CAD build for the part. Positions are in the model's coordinates, mm. A direction names the side the tool comes from. Give positions to 0.01 mm unless a question says otherwise; leave off trailing zeros. Order: outer loops, then holes, each group sorted by start corner. A loop starts at its lowest first (then second) coordinate and runs counter-clockwise, first axis right, second up. Notation, with made-up numbers: (53, -17.75) -> (112, -17.75) arc R9 ccw to (112, -0.75) -> close; hole circle Ø3 at (-33.75, -24). An arc over 180 degrees is marked (long way). Answer as CSV lines item,"result".
Autodesk Inventor part; units mm, degrees
ref_plane "YZ Plane" through (0, 0, 0) normal (1, 0, 0) x (0, 1, 0)
ref_plane "XZ Plane" through (0, 0, 0) normal (0, 1, 0) x (-1, 0, 0)
ref_plane "XY Plane" through (0, 0, 0) normal (0, 0, 1) x (1, 0, 0)
sketch "Esboço1" plane through (0, 0, 0) normal (0, 1, 0) x (-1, 0, 0)
  line L0 (0, 0) -> (0, -16)
  line L1 (0, -16) -> (-34.5, -16)
  line L2 (-34.5, -16) -> (-34.5, 0)
  line L3 (-34.5, 0) -> (0, 0)
  line L4 (-3.5, -14.5) -> (-16.5, -14.5)
  line L5 (-16.5, -14.5) -> (-16.5, -1.5)
  line L6 (-16.5, -1.5) -> (-3.5, -1.5)
  line L7 (-18, -14.5) -> (-33, -14.5)
  line L8 (-33, -14.5) -> (-33, -1.5)
  line L9 (-33, -1.5) -> (-18, -1.5)
  line L10 (-18, -1.5) -> (-18, -14.5)
  line L11 (-3.5, -14.5) -> (-3.5, -12)
  line L12 (-3.5, -12) -> (-1.5, -12)
  line L13 (-1.5, -12) -> (-1.5, -4)
  line L14 (-1.5, -4) -> (-3.5, -4)
  line L15 (-3.5, -4) -> (-3.5, -1.5)
  point P0 (-34.5, -8)
  dimension "d0" = 13
  dimension "d1" = 13
  dimension "d2" = 15
  dimension "d3" = 13
  dimension "d4" = 8
  dimension "d5" = 2.5
  dimension "d6" = 1.5
  dimension "d7" = 1.5
  dimension "d8" = 2
  dimension "d9" = 1.5
  dimension "d10" = 1.5
  dimension "d11" = 1.5
extrude "Extrusão1" add sketch "Esboço1" along normal blind 1.5 contours L4 L5 L6 L15 L14 L13 L12 L11 | L7 L8 L9 L10
extrude "Extrusão2" add sketch "Esboço1" along normal blind 20
sketch "Esboço2" plane through (0, 0, -16) normal (-1, 0, 0) x (0, 0, 1)
  line L0 (12, 20) -> (4, 20)
  line L1 (8, 20) -> (8, 0)
  line L2 (0, 0) -> (0, 20)
  circle A0 centre (5.45, 8) radius 0.5
  circle A1 centre (10.55, 8) radius 0.5
  line L3 (0, 0) -> (16, 0)
  dimension "d23" = 8
extrude "Extrusão3" cut sketch "Esboço2" against normal blind 10
sketch "Esboço3" plane through (34.5, 0, 0) normal (1, 0, 0) x (0, 0, -1)
  line L0 (0, 20) -> (16, 20)
  line L1 (8, 20) -> (8, 0)
  circle A0 centre (6.75, 8) radius 0.5
  circle A1 centre (9.25, 8) radius 0.5
  line L2 (0, 0) -> (16, 0)
  line L3 (11, 16) -> (11, 8)
  line L4 (11, 8) -> (5, 8)
  line L5 (5, 8) -> (5, 16)
  circle A2 centre (5, 12) radius 1.5
  circle A3 centre (11, 12) radius 1.5
  dimension "d26" = 1
  dimension "d27" = 1
  dimension "d28" = 8
  dimension "d29" = 8
  dimension "d30" = 1.25
  dimension "d31" = 1.25
  dimension "d78" = 3
  dimension "d79" = 3
  dimension "d80" = 3
  dimension "d81" = 3
extrude "Extrusão4" cut sketch "Esboço3" against normal blind 10 contours L4 A0 | A1 L4 | L4 A1 | A0 L4
sketch "Esboço4" plane through (18, 1.5, -14.5) normal (1, 0, 0) x (0, 0, -1)
  line L0 (-14.5, -1.5) -> (1.5, -1.5)
  line L1 (-6.5, -1.5) -> (-6.5, 18.5)
  line L2 (0, 18.5) -> (-13, 18.5)
  circle A0 centre (-6.5, 6.5) radius 2.5
  line L3 (0, 0) -> (-13, 0)
  dimension "d40" = 5
  dimension "d42" = 6.5
extrude "Extrusão5" cut sketch "Esboço4" against normal blind 10
sketch "Esboço6" plane through (0, 20, 0) normal (0, 1, 0) x (1, 0, 0)
  line L0 (0, 0) -> (34.5, 0)
  line L1 (0, 0) -> (16.5, 0)
  line L2 (0, 0) -> (16.5, 0) construction
  line L3 (16.5, 14.5) -> (16.5, 1.5)
  line L4 (16.5, 0) -> (16.5, 1.5)
  line L5 (16.5, 1.5) -> (3.5, 1.5)
  line L6 (16.5, 1.5) -> (3.5, 1.5)
  line L7 (3.5, 1.5) -> (3.5, 4)
  line L8 (3.5, 1.5) -> (3.5, 4)
  line L9 (3.5, 4) -> (1.5, 4)
  line L10 (3.5, 4) -> (1.5, 4)
  line L11 (1.5, 4) -> (1.5, 12)
  line L12 (1.5, 12) -> (3.5, 12)
  line L13 (1.5, 12) -> (3.5, 12)
  line L14 (3.5, 12) -> (3.5, 14.5)
  line L15 (3.5, 12) -> (3.5, 14.5)
  line L16 (3.5, 14.5) -> (16.5, 14.5)
  line L17 (3.5, 14.5) -> (16.5, 14.5)
  line L18 (16.5, 14.5) -> (16.5, 16)
  line L19 (34.5, 16) -> (0, 16)
  line L20 (0, 16) -> (0, 0)
  line L21 (0, 16.0004) -> (0, 0)
  dimension "d66" = 16.5
  dimension "d67" = 0
extrude "Extrusão8" add sketch "Esboço6" along normal blind 3.5 contours L20 L19 L18 L16 L14 L12 L11 L9 L7 L5 L4 L0
sketch "Sketch8" plane through (0, 23.5, 0) normal (0, 1, 0) x (1, 0, 0)
  line L0 (3.5, 1.5) -> (16.5, 1.5)
  line L1 (6, 1.5) -> (6, -0.5)
  line L2 (6, -0.5) -> (14, -0.5)
  line L3 (14, -0.5) -> (14, 1.5)
  line L4 (16.5, 1.5) -> (14, 1.5)
  line L5 (3.5, 1.5) -> (3.5, -2)
  line L6 (3.5, -2) -> (16.5, -2)
  line L7 (16.5, -2) -> (16.5, 1.5)
  line L8 (0, 0) -> (34.5, 0)
  point P0 (6, 0)
  point P1 (14, 0)
  dimension "d86" = 8
  dimension "d87" = 2.5
  dimension "d88" = 2
  dimension "d89" = 2
  dimension "d90" = 3.5
extrude "Extrusion12" add sketch "Sketch8" against normal up to surface (23.5 mm away) contours L0 L1 L8 L5 | L8 L1 L2 L3 L7 L6 L5 | L0 L7 L8 L3
extrude "Extrusion13" cut sketch "Sketch8" against normal blind 22 contours L0 L3 L8 L1
sketch "Sketch9" plane through (0, 23.5, 0) normal (0, 1, 0) x (1, 0, 0)
  line L0 (34.5, 16) -> (0, 16)
  line L1 (0, 0) -> (3.5, 0)
  line L2 (0, 16) -> (1.5, 16)
  line L3 (1.5, 16) -> (1.5, 0)
  line L4 (1.5, 0) -> (0, 0)
  line L5 (0, 0) -> (0, 16)
  line L6 (3.5, 12) -> (1.5, 12)
  line L7 (3.5, 1.5) -> (3.5, 4)
  line L8 (3.5, 12) -> (3.5, 4)
  dimension "d95" = 1.5
extrude "Extrusion14" cut sketch "Sketch9" against normal through all
sketch "Sketch10" plane through (0, 23.5, 0) normal (0, 1, 0) x (1, 0, 0)
  line L0 (3.5, 14.5) -> (3.5, 12)
  line L1 (1.5, 12) -> (1.5, 4)
  line L2 (3.5, 12) -> (1.5, 12)
  line L3 (1.5, 12) -> (1.5, 4)
  line L4 (1.5, 4) -> (3.5, 4)
  line L5 (3.5, 4) -> (3.5, 12)
  point P0 (0, 0)
extrude "Extrusion15" add sketch "Sketch10" against normal up to surface (22 mm away)
sketch "Sketch11" plane through (0, 0, 0) normal (0, -1, 0) x (1, 0, 0)
  line L0 (6, 0) -> (14, 0)
  line L1 (6, 0.5) -> (14, 0.5)
  line L2 (6, 0) -> (14, 0)
  line L3 (14, 0) -> (14, 0.5)
  line L4 (14, 0.5) -> (6, 0.5)
  line L5 (6, 0.5) -> (6, 0)
  point P0 (0, 0)
extrude "Extrusion16" add sketch "Sketch11" against normal blind 1.5
sketch "Sketch12" plane through (0, 23.5, 0) normal (0, 1, 0) x (1, 0, 0)
  line L0 (1.5, 16) -> (1.5, 0)
  line L1 (3.5, -2) -> (3.5, 0)
  line L2 (1.5, 0) -> (3.5, 0)
  line L3 (3.5, 0) -> (3.5, -2)
  line L4 (3.5, -2) -> (1.5, -2)
  line L5 (1.5, -2) -> (1.5, 0)
  point P0 (0, 0)
extrude "Extrusion17" add sketch "Sketch12" against normal up to surface (23.5 mm away)
sketch "Sketch13" plane through (16.5, 0, 2) normal (0, 0, 1) x (1, 0, 0)
  line L0 (-13, 23.5) -> (0, 23.5)
  line L1 (-6.5, 23.5) -> (-6.5, 0)
  circle A0 centre (-3.95, 8) radius 0.75
  circle A1 centre (-9.05, 8) radius 0.75
  line L2 (0, 0) -> (-15, 0)
  line L3 (0, 23.5) -> (0, 0)
  point P0 (-16.5, 0)
  dimension "d104" = 1.5
  dimension "d105" = 1.5
  dimension "d106" = 8
  dimension "d107" = 8
  dimension "d108" = 6.5
  dimension "d109" = 2.55
  dimension "d110" = 2.55
extrude "Extrusion18" cut sketch "Sketch13" against normal blind 10 contours A0 | A1
properties part number "Base_3DPrint"
1) Band-saw the part on B-B, the plane y = 16.5. Write the cut outline in (x, z), then the cut area to 3 significant figures.
Data:
outline,"(1.5, -16) -> (34.5, -16) -> (34.5, 0) -> (16.5, 0) -> (16.5, 2) -> (1.5, 2) -> close; hole (3.5, -14.5) -> (16.5, -14.5) -> (16.5, -1.5) -> (14, -1.5) -> (14, 0.5) -> (6, 0.5) -> (6, -1.5) -> (3.5, -1.5) -> close; hole (18, -14.5) -> (33, -14.5) -> (33, -1.5) -> (18, -1.5) -> close"
area,"178 mm2"
2) Pin check, flat tips, straight feed: P1, Ø5, axis at x = 28, z = -1, coming from the +Y side; P2, Ø5, axis at x = 9, z = -2.5, coming from the +Y side; P3, Ø1.6, axis at y = 21.5, z = -15, coming from the +X side. Stop position of each tip, or through.
Data:
P1,"stops at y = 20"
P2,"stops at y = 1.5"
P3,"stops at x = 16.5"
3) Band-saw the part on A-A, the plane x = 7.45. Write the cut outline in (y, z).
Data:
outline,"(0, -16) -> (23.5, -16) -> (23.5, -14.5) -> (1.5, -14.5) -> (1.5, 0.5) -> (7.25, 0.5) -> (7.25, 2) -> (0, 2) -> close; (8.75, 0.5) -> (23.5, 0.5) -> (23.5, 2) -> (8.75, 2) -> close"
4) Band-saw the part on C-C, the plane z = -8. Write the cut outline in (x, y), then the cut area to 4 significant figures.
Data:
outline,"(1.5, 0) -> (34.5, 0) -> (34.5, 20) -> (33, 20) -> (33, 1.5) -> (18, 1.5) -> (18, 5.5) -> (16.5, 5.5) -> (16.5, 1.5) -> (3.5, 1.5) -> (3.5, 23.5) -> (1.5, 23.5) -> close; (16.5, 10.5) -> (18, 10.5) -> (18, 20) -> (16.5, 20) -> close"
area,"141.5 mm2"
5) Band-saw the part on D-D, the plane x = 27. Write the cut outline in (y, z), then the cut area to 3 significant figures.
Data:
outline,"(0, -16) -> (20, -16) -> (20, -14.5) -> (1.5, -14.5) -> (1.5, -1.5) -> (20, -1.5) -> (20, 0) -> (0, 0) -> close"
area,"79.5 mm2"
6) Which spindle directions (+Z, -Z, +X, -X, +Y, -Y) get a long thin tool onto all of the face, cutting with end or side? Do faces 1 (the flat face through (15, 12, -1.5)), 2 (the cylindrical face through (17.26, 5.78, -9.15)), 3 (the flat face through (26, 20, -15)). Say none if no direction does.
Data:
face 1,"+Y"
face 2,"none"
face 3,"+Z, -Z, +X, +Y"
7) Pull direction Y, two halves, no side cores. Call faces 4 (the cylindrical face through (11.8, 8, 1.3)), 5 (the cylindrical face through (33.76, 7.556, -6.981)), 6 (the flat face through (3, 23.5, -6)), 7 (the flat face through (18, 0, -7)): pulls with the +Y half, pulls with the -Y half, needs draft (parallel to the pull), parting line crosses it, or undercut.
Data:
face 4,"undercut"
face 5,"undercut"
face 6,"pulls with the +Y half"
face 7,"pulls with the -Y half"
8) Wall check: line 1 along X through (y, z) = (14, -2.25); line 2 along Y through (x, z) = (17.55, -8); line 3 along Z through (x, y) = (33.4, 8). Give the ranges that are in metal, low to high. Write a range as [from, to].
Data:
line 1,"x = [1.5, 3.5], [16.5, 18], [33, 34.5]"
line 2,"y = [0, 5.5], [10.5, 20]"
line 3,"z = [-16, -9.75], [-8.75, -7.25], [-6.25, 0]"
